Check sheet for the drawn part. Datum: minimum x, y, z corner. Units: mm. A direction names the side the tool comes from. Give positions to 0.01 mm unless a question says otherwise; leave off trailing zeros. Order: outer loops, then holes, each group sorted by start corner. A loop starts at its lowest first (then second) coordinate and runs counter-clockwise, first axis right, second up.
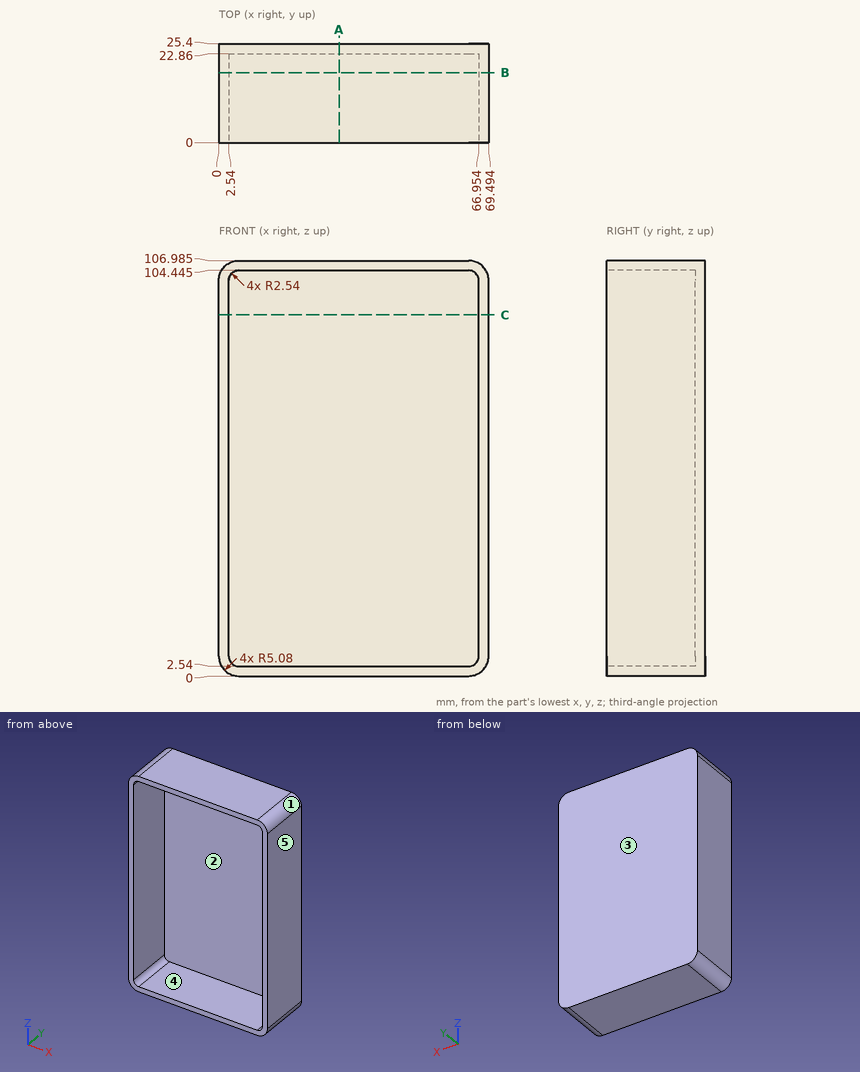
Item 1: Sectioned sample at C-C (z = 93). Enter the section's corners in (x, y) (1 decimal).
Reported:
outline: (0, 0) - (2.5, 0) - (2.5, 22.9) - (67, 22.9) - (67, 0) - (69.5, 0) - (69.5, 25.4) - (0, 25.4) - close
Item 2: Scan lines: L1, parallel to X at y = 22.75, z = 51 (1 decimal); L2, parallel to Z at x = 39.5, y = 9.5 (1 decimal); L3, parallel to Y at x = 66, z = 60. Record each from-to range of solid material in increasing order.
Reported:
L1: x = 0 to 2.5, 67 to 69.5
L2: z = 0 to 2.5, 104.4 to 107
L3: y = 22.86 to 25.4
Item 3: Sectioned sample at B-B (y = 18). Enter the section's corners in (x, z) (1 decimal).
Reported:
outline: (0, 5.1) arc R5.1 ccw to (5.1, 0) - (64.4, 0) arc R5.1 ccw to (69.5, 5.1) - (69.5, 101.9) arc R5.1 ccw to (64.4, 107) - (5.1, 107) arc R5.1 ccw to (0, 101.9) - close; hole (2.5, 5.1) arc R2.5 ccw to (5.1, 2.5) - (64.4, 2.5) arc R2.5 ccw to (67, 5.1) - (67, 101.9) arc R2.5 ccw to (64.4, 104.4) - (5.1, 104.4) arc R2.5 ccw to (2.5, 101.9) - close
Item 4: Gauge pin test, flat ends, axial feed: pin 1 (3 mm diameter, centred on x = 13, z = 77.5, fed in from -Y); pin 2 (7 mm diameter, centred on y = 9.5, z = 48.5, fed in from -X). Record the tip position at first contact, or that the pin passes through.
Reported:
pin 1: stops at y = 22.86
pin 2: stops at x = 0
Item 5: Set-up check for the marked faces 4 and 5: record each of +Z, -Z, +X, -X, +Y, -Y from which the full face is reachable in a straight line by a thin tool's end or side.
Reported:
face 4: -Y
face 5: +Z, -Z, +X, +Y, -Y
Item 6: Sectioned sample at A-A (x = 31). Enter the section's corners in (y, z) (1 decimal).
Reported:
outline: (0, 0) - (25.4, 0) - (25.4, 107) - (0, 107) - (0, 104.4) - (22.9, 104.4) - (22.9, 2.5) - (0, 2.5) - close
Item 7: Draft check along Z on the marked faces 1, 2 and 3. Enter one of: released by +Z, released by -Z, zero draft, split by the parting line, or undercut.
Reported:
face 1: released by +Z
face 2: undercut
face 3: zero draft
